Autodesk Fusion 360 part; units mm, degrees
sketch "Boceto1" plane through (0, 0, 0) normal (0, 1, 0) x (1, 0, 0)
  line L0 (-30, 20) -> (160, 20)
  line L1 (160, 20) -> (160, -75)
  line L2 (160, -75) -> (-30, -75)
  line L3 (-30, -75) -> (-30, 20)
  dimension "d1" = 190
  dimension "d2" = 95
extrude "Extruir1" add sketch "Boceto1" along normal blind 5
sketch "Boceto2" plane through (0, 0, 0) normal (0, -1, 0) x (1, 0, 0)
  line L0 (160, 75) -> (-30, 75)
  line L1 (-30, 75) -> (-30, -20)
  line L2 (-30, -20) -> (160, -20)
  line L3 (160, -20) -> (160, 75)
  line L4 (-30, 27.5) -> (5, 27.5)
  line L5 (65, 52.5) -> (5, 52.5)
  line L6 (125, 27.5) -> (125, 2.5)
  line L7 (5, 52.5) -> (125, 52.5)
  line L8 (125, 52.5) -> (125, 2.5)
  line L9 (125, 2.5) -> (5, 2.5)
  line L10 (5, 2.5) -> (5, 52.5)
  point P0 (65, 27.5)
  dimension "d5" = 47.5
  dimension "d6" = 95
  dimension "d7" = 25
  dimension "d8" = 60
  dimension "d9" = 60
  dimension "d10" = 25
extrude "Extruir2" add sketch "Boceto2" along normal blind 50 contours L5 L6 L7 L8 L9 L10
sketch "Boceto3" plane through (125, 0, 0) normal (1, 0, 0) x (0, 0, -1)
  line L0 (-2.5, 0) -> (-52.5, 0)
  line L1 (-52.5, 0) -> (-52.5, -50)
  line L2 (-52.5, -50) -> (-2.5, -50)
  line L3 (-2.5, -50) -> (-2.5, 0)
  line L4 (-52.5, -50) -> (-27.5, -50)
  line L5 (-27.5, -50) -> (-27.5, -46)
  circle A0 centre (-27.5, -33.525) radius 12.475
  dimension "d13" = 25
  dimension "d14" = 4
  dimension "d15" = 24.95
extrude "Extruir3" cut sketch "Boceto3" against normal blind 150 contours A0
sketch "Boceto4" plane through (125, 0, 0) normal (1, 0, 0) x (0, 0, -1)
  circle A0 centre (-27.5, -33.525) radius 12.475
  line L0 (-2.5, 0) -> (-52.5, 0)
  line L1 (-52.5, 0) -> (-52.5, -50)
  line L2 (-52.5, -50) -> (-2.5, -50)
  line L3 (-2.5, -50) -> (-2.5, 0)
  line L4 (-27.5, -33.525) -> (-18.5, -33.525)
  line L5 (-18.5, -33.525) -> (-18.5, -26.025)
  line L6 (-18.5, -26.025) -> (-11.5, -26.025)
  line L7 (-11.5, -26.025) -> (-11.5, -41.025)
  line L8 (-11.5, -41.025) -> (-18.5, -41.025)
  line L9 (-18.5, -41.025) -> (-18.5, -26.025)
  dimension "d18" = 9
  dimension "d19" = 7.5
  dimension "d20" = 7
  dimension "d21" = 15
extrude "Extruir4" cut sketch "Boceto4" against normal blind 180 contours A0 L6 L7 L8
fillet "Empalme1" radius 25 2 edges at (65, -50, 2.5) (65, -50, 52.5)
sketch "Boceto5" plane through (0, 0, 0) normal (0, 0, 1) x (1, 0, 0)
  line L0 (64.5, -25) -> (64.5, -45)
  line L1 (68.5, -25) -> (68.5, -45)
  line L2 (65.5, -25) -> (65.5, -5)
  line L3 (64.5, -5) -> (64.5, -25)
  line L4 (64.5, -45) -> (54.5, -45)
  line L5 (54.5, -45) -> (64.5, -45)
  line L6 (64.5, -45) -> (64.5, -5)
  line L7 (64.5, -5) -> (54.5, -5)
  line L8 (54.5, -5) -> (54.5, -45)
  line L9 (68.5, -45) -> (75.5, -45)
  line L10 (75.5, -45) -> (65.5, -45)
  line L11 (65.5, -45) -> (65.5, -5)
  line L12 (65.5, -5) -> (75.5, -5)
  line L13 (75.5, -5) -> (75.5, -45)
  line L14 (54.5, -40.8747) -> (75.5, -40.8747)
  line L15 (54.5, -23.0491) -> (75.5, -23.0491)
  dimension "d33" = 20
  dimension "d35" = 20
  dimension "d36" = 10
  dimension "d37" = 7
  dimension "d38" = 10
extrude "Extruir5" cut sketch "Boceto5" along normal blind 31 contours L0 L3 L6 L8 L14 L15 | L2 L11 L13 L14 L15
sketch "Boceto6" plane through (0, 0, 11.5) normal (0, 0, 1) x (1, 0, 0)
  line L0 (54.5, -40.8747) -> (54.5, -26.025)
  line L1 (54.5, -26.025) -> (5, -26.025)
  line L2 (5, -26.025) -> (5, -41.025)
  line L3 (5, -41.025) -> (125, -41.025)
  line L4 (125, -41.025) -> (125, -26.025)
  line L5 (125, -26.025) -> (75.5, -26.025)
  line L6 (75.5, -26.025) -> (75.5, -40.8747)
  line L7 (75.5, -40.8747) -> (65.5, -40.8747)
  line L8 (65.5, -40.8747) -> (65.5, -26.025)
  line L9 (65.5, -26.025) -> (64.5, -26.025)
  line L10 (64.5, -26.025) -> (64.5, -40.8747)
  line L11 (64.5, -40.8747) -> (54.5, -40.8747)
  line L12 (64.5, -48.0409) -> (65.5441, -48.0409)
  line L13 (65.5441, -48.0409) -> (65.5441, -10.5894)
  line L14 (65.5441, -10.5894) -> (64.5, -10.5894)
  line L15 (64.5, -10.5894) -> (64.5, -48.0409)
extrude "Extruir6" add sketch "Boceto6" along normal blind 30 contours L3 L7 L8 L9 L10 L13 L15 | L7 L8 L9 L13 L14 L15 | L3 L12 L13 L15
sketch "Boceto7" plane through (65.5441, 0, 0) normal (1, 0, 0) x (0, 0, -1)
  arc A0 (-17.7987, -48.0409) -> (-11.5, -44.2094) centre (-27.5, -25) ccw
  line L0 (-17.7987, -48.0409) -> (-11.5, -48.0409)
  line L1 (-11.5, -48.0409) -> (-11.5, -44.2094)
  arc A1 (-41.5, -45.7123) -> (-37.2013, -48.0409) centre (-27.5, -25) ccw
  line L2 (-41.5, -45.7123) -> (-41.5, -48.0409)
  line L3 (-41.5, -48.0409) -> (-37.2013, -48.0409)
extrude "Extruir7" cut sketch "Boceto7" against normal blind 9
sketch "Boceto8" plane through (125, 0, 0) normal (1, 0, 0) x (0, 0, -1)
  line L0 (-11.5, -41.025) -> (-17.5313, -41.025)
  arc A0 (-17.5313, -26.025) -> (-17.5313, -41.025) centre (-27.5, -33.525) ccw
  line L1 (-17.5313, -26.025) -> (-11.5, -26.025)
  line L2 (-11.5, -26.025) -> (-11.5, -41.025)
  arc A1 (-52.5, -25) -> (-2.5, -25) centre (-27.5, -25) ccw
  line L3 (-2.5, -25) -> (-2.5, 0)
  line L4 (-2.5, 0) -> (-52.5, 0)
  line L5 (-52.5, 0) -> (-52.5, -25)
  line L6 (-27.5, -33.525) -> (-27.5, -48)
sketch "Boceto9" plane through (0, 5, 0) normal (0, 1, 0) x (-1, 0, 0)
  line L0 (30, 75) -> (-160, 75)
  line L1 (-160, 75) -> (-160, -20)
  line L2 (-160, -20) -> (30, -20)
  line L3 (30, -20) -> (30, 75)
  line L4 (30, 75) -> (30, 27.5)
  line L5 (30, 27.5) -> (-65, 27.5)
  line L6 (-65, 27.5) -> (-102.5, 27.5)
  line L7 (-102.5, 27.5) -> (-102.5, 44.5)
  line L8 (-102.5, 44.5) -> (-27.5, 44.5)
  line L9 (-27.5, 44.5) -> (-27.5, 10.5)
  line L10 (-27.5, 10.5) -> (-102.5, 10.5)
  line L11 (-102.5, 10.5) -> (-102.5, 44.5)
  dimension "d47" = 47.5
  dimension "d48" = 95
  dimension "d49" = 37.5
  dimension "d50" = 17
  dimension "d51" = 34
  dimension "d52" = 75
extrude "Extruir8" cut sketch "Boceto9" against normal blind 10 contours L5 L6 L9 L10 L11 | L5 L6 L7 L8 L9 L11
sketch "Boceto10" plane through (0, 5, 0) normal (0, 1, 0) x (-1, 0, 0)
  line L0 (-27.5, 44.5) -> (-27.5, 10.5)
  line L1 (-27.5, 10.5) -> (-102.5, 10.5)
  line L2 (-102.5, 10.5) -> (-102.5, 44.5)
  line L3 (-102.5, 44.5) -> (-27.5, 44.5)
  line L4 (30, 75) -> (-160, 75)
  line L5 (-160, 75) -> (-160, -20)
  line L6 (-160, -20) -> (30, -20)
  line L7 (30, -20) -> (30, 75)
  line L8 (-27.5, 44.5) -> (-16.0562, 44.5)
  line L9 (-16.0562, 44.5) -> (-16.0562, 38.0888)
  line L10 (-16.0562, 38.0888) -> (-27.5, 38.0888)
  line L11 (-27.5, 38.0888) -> (-27.5, 44.5)
  line L12 (-27.5, 10.5) -> (-16.0562, 10.5)
  line L13 (-16.0562, 10.5) -> (-16.0562, 16.8458)
  line L14 (-16.0562, 16.8458) -> (-27.5, 16.8458)
  line L15 (-27.5, 16.8458) -> (-27.5, 10.5)
extrude "Extruir9" cut sketch "Boceto10" against normal blind 10 contours L0 L8 L9 L10 L11 | L0 L12 L13 L14 L15
fillet "Empalme2" radius 10 2 edges at (27.5, 0, 16.8458) (27.5, 0, 38.0888)
sketch "Boceto11" plane through (0, 5, 0) normal (0, 1, 0) x (-1, 0, 0)
  arc A0 (-17.5, 38.0888) -> (-27.5, 28.0888) centre (-17.5, 28.0888) ccw
  line L0 (-27.5, 28.0888) -> (-27.5, 26.8458)
  arc A1 (-27.5, 26.8458) -> (-17.5, 16.8458) centre (-17.5, 26.8458) ccw
  line L1 (-17.5, 16.8458) -> (-16.0562, 16.8458)
  line L2 (-16.0562, 16.8458) -> (-16.0562, 10.5)
  line L3 (-16.0562, 10.5) -> (-102.5, 10.5)
  line L4 (-102.5, 10.5) -> (-102.5, 44.5)
  line L5 (-102.5, 44.5) -> (-16.0562, 44.5)
  line L6 (-16.0562, 44.5) -> (-16.0562, 38.0888)
  line L7 (-16.0562, 38.0888) -> (-17.5, 38.0888)
  line L8 (30, 75) -> (-160, 75)
  line L9 (-160, 75) -> (-160, -20)
  line L10 (-160, -20) -> (30, -20)
  line L11 (30, -20) -> (30, 75)
Design review of the part built by this model. Coordinates are the model's own, in mm. A direction names the side the tool comes from. Round coordinates to 2 decimals unless told otherwise and drop trailing zeros. Write each loop counter-clockwise with the first axis right and the second up, starting at its lowest first coordinate (ties: lowest second). Pieces come first, ordered by that corner, then holes. Notation, with made-up numbers: (32.25, 68) -> (89.25, 68) arc R18 ccw to (89.25, 103) -> close; hole circle Ø1 at (37, 31). An arc over 180 degrees is marked (long way). One line per question, with ' | ' between items.
(1) Take a section at B-B, the plane y = -31. State the section outline as (x, z) points.
Result sheet:
outline: (5, 3.23) -> (54.5, 3.23) -> (54.5, 11.5) -> (5, 11.5) -> close; (5, 39.72) -> (64.5, 39.72) -> (64.5, 3.23) -> (65.5, 3.23) -> (65.5, 11.5) -> (65.54, 11.5) -> (65.54, 39.72) -> (125, 39.72) -> (125, 51.77) -> (5, 51.77) -> close; (75.5, 3.23) -> (125, 3.23) -> (125, 11.5) -> (75.5, 11.5) -> close
(2) Draft analysis for pull direction Y (two halves, no side actions). For faces 1 (the cylindrical face through (64.16, -42.484, 9.628)), 2 (the flat face through (64.5, -33, 21)), 3 (the flat face through (66, 2, 75)), state which applies: released by +Y, released by -Y, zero draft, split by the parting line, or undercut.
Result sheet:
face 1: released by -Y | face 2: undercut | face 3: zero draft
(3) Wall thickness on line 1 (X direction, y = -30.5, z = 10.5); line 2 (Y direction, x = 92, z = 27); line 3 (X direction, y = -1.5, z = 44): over which ranges is each line inside the solid? List them lowest first. Write a range as [from, to].
Result sheet:
line 1: [5, 54.5], [64.5, 65.5], [75.5, 125] | line 2: [-50, -45.99], [-21.06, -5] | line 3: [5, 16.06], [102.5, 125]
(4) Machinability: for faces 4 (the flat face through (5, -19, 27)), 5 (the flat face through (66, -12, 52.5)), 6 (the flat face through (66, -12, 2.5)), 7 (the flat face through (59, 0, 10.5)), which of the approach directions +Z, -Z, +X, -X, +Y, -Y give a long, thin tool a straight path to every point of the face, cutting with its end or side? Answer none if there is none.
Result sheet:
face 4: +Z, -Z, -X, -Y | face 5: +Z, +X, -X, -Y | face 6: -Z, +X, -X, -Y | face 7: +Y
(5) Take a section at A-A, the plane x = 100.5. State the section outline as (y, z) points (3 decimals).
Result sheet:
outline: (-50, 27.495) arc R24.995 ccw to (-25.005, 2.5) -> (0, 2.5) -> (0, -20) -> (5, -20) -> (5, 10.5) -> (-5, 10.5) -> (-5, 44.5) -> (5, 44.5) -> (5, 75) -> (0, 75) -> (0, 52.5) -> (-25.005, 52.5) arc R24.995 ccw to (-50, 27.505) -> close; hole (-41.025, 11.5) -> (-26.025, 11.5) -> (-26.025, 17.531) arc R12.475 ccw (long way) to (-41.025, 17.531) -> close
(6) Take a section at C-C, the plane z = -7.5. State the section outline as (x, y) points.
Result sheet:
outline: (-30, 0) -> (160, 0) -> (160, 5) -> (-30, 5) -> close
(7) Take a section at D-D, the plane x = 131.5. State the section outline as (y, z) points, and give its area (3 significant figures).
Result sheet:
outline: (0, -20) -> (5, -20) -> (5, 75) -> (0, 75) -> close | area: 475 mm2
(8) Insertion check: P1, Ø1, axis at y = -1.5, z = 27.5, coming from the +X side; P2, Ø5, axis at x = 51.5, z = 49.5, coming from the -Y side; P3, Ø6, axis at y = -7, z = 24.5, coming from the -X side. Each pin has a flat end and moves straight along its axis. Give the tip position at first contact, or say it passes through.
Result sheet:
P1: x = 125 | P2: y = -40.65 | P3: x = 5
